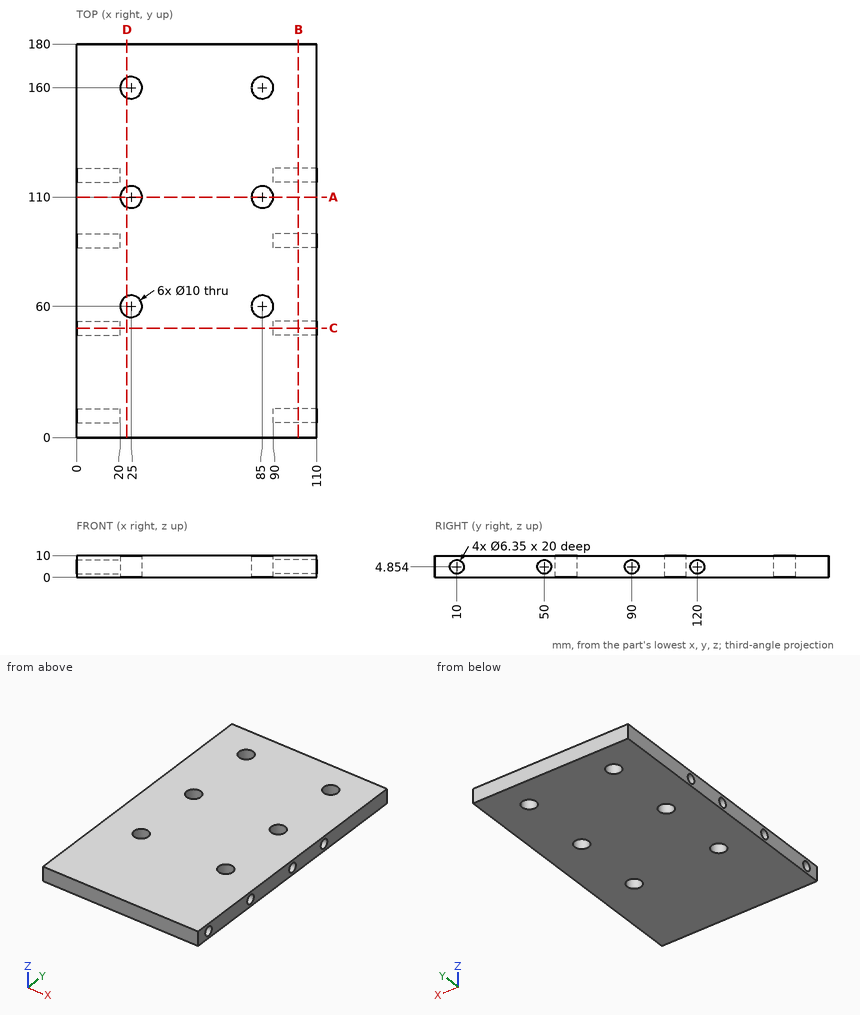
Geometry: see drawing. Coordinates: mm, zero at the bounding-box minimum. Coordinates: 2 decimals unless noted, no trailing zeros. Order: outer loops, then holes, each group sorted by start corner. A loop starts at its lowest first (then second) coordinate and runs counter-clockwise, first axis right, second up. Notation, with made-up numbers: M 45,-30 L 50,-30 A10 cw 50,-17 Z; hole C 83.25,81.5 d2. An arc over 180 degrees is marked long. Write item = value, one per line. Start each with the question number.
(1) Section C-C on y = 50. Output: boundary loops of the cut face in (x, z), and give its area (3 significant figures).
(2) Line query: line 1 along X through (y, z) = (160.5, 3.25) (1 decimal); line 2 along Y through (x, z) = (25.5, 1.75) (1 decimal); line 3 along Y through (x, z) = (93.5, 5). Output: solid intervals per line, ascending. Write a range as [from, to].
(3) First-contact query: P1, Ø5, axis at y = 10, z = 4.85, coming from the +X side; P2, Ø11.5, axis at x = 25, y = 60, coming from the -Z side; P3, Ø9, axis at x = 25, y = 160, coming from the +Z side; P4, Ø3, axis at y = 119.5, z = 4.5, coming from the -X side. Flat tips, straight axial feed; report the tip coordinate or a pass-through.
(4) Section A-A on y = 110. Output: boundary loops of the cut face in (x, z), and give its area (3 significant figures).
(5) Section B-B on x = 101.5. Give the number of separate pieces and of enclosed holes in the cut face, and give its area (3 significant figures).
(6) Section D-D on x = 23. Output: boundary loops of the cut face in (y, z), and give its area (4 significant figures).
Result set:
q1.outline = M 0,0 L 110,0 L 110,1.68 L 90,1.68 L 90,8.03 L 110,8.03 L 110,10 L 0,10 L 0,8.03 L 20,8.03 L 20,1.68 L 0,1.68 Z
q1.area = 846 mm²
q2.line_1 = [0, 20], [30, 80], [90, 110]
q2.line_2 = [0, 55], [65, 105], [115, 155], [165, 180]
q2.line_3 = [0, 6.83], [13.17, 46.83], [53.17, 86.83], [93.17, 116.83], [123.17, 180]
q3.P1 = 90
q3.P2 = 0
q3.P3 = through
q3.P4 = 20
q4.outline = M 0,0 L 20,0 L 20,10 L 0,10 Z; M 30,0 L 80,0 L 80,10 L 30,10 Z; M 90,0 L 110,0 L 110,10 L 90,10 Z
q4.area = 900 mm²
q5.separate_pieces = 1
q5.enclosed_holes = 4
q5.area = 1,670 mm²
q6.outline = M 0,0 L 55.42,0 L 55.42,10 L 0,10 Z; M 64.58,0 L 105.42,0 L 105.42,10 L 64.58,10 Z; M 114.58,0 L 155.42,0 L 155.42,10 L 114.58,10 Z; M 164.58,0 L 180,0 L 180,10 L 164.58,10 Z
q6.area = 1,525 mm²
